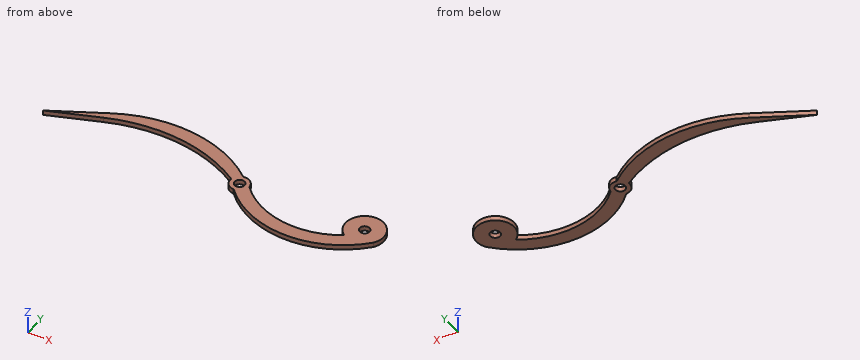
from build123d import *

# Parameters (mm, degrees)
F0_R     = 1.651
F1_DEPTH = 1.6002


with BuildPart() as f1:
    # F0 (on Top) → F1 (new body)
    with BuildSketch(Plane.XY):
        with BuildLine():
            ThreePointArc((-3.774051, -5.106764), (-21.934308, -8.777509), (-38.227296, 0.043366))
            ThreePointArc((-38.227296, 0.043366), (-39.403324, 2.466965), (-42.018165, 3.114637))
            ThreePointArc((-42.018165, 3.114637), (-64.733422, 13.156228), (-89.188089, 8.82198))
            Line((-89.188089, 8.82198), (-106.5022, 0))
            Line((-106.5022, 0), (-90.018623, 5.999531))
            ThreePointArc((-90.018623, 5.999531), (-66.625194, 8.705331), (-44.525194, 0.571215))
            ThreePointArc((-44.525194, 0.571215), (-43.86651, -2.001703), (-41.483321, -3.173958))
            ThreePointArc((-41.483321, -3.173958), (-18.287164, -13.645991), (5.147266, -3.718622))
            ThreePointArc((5.147266, -3.718622), (-0.976301, 6.274499), (-3.774051, -5.106764))
        make_face()
        with Locations((-41.402, 0)):
            Circle(F0_R, mode=Mode.SUBTRACT)
        Circle(F0_R, mode=Mode.SUBTRACT)
    extrude(amount=F1_DEPTH)


solid = f1.part
Geometry check sheet. Reference: the model listing, model coordinates, mm. Coordinates: 2 decimals unless noted, no trailing zeros. Loops run counter-clockwise (first coordinate to the right, second up) from the corner with the lowest first, then second, coordinate; pieces in that order, holes last. Notation, with made-up numbers: (87.25, 22.25) - (138.25, 22.25) arc R32 cw to (138.25, 49.25) - close; hole circle Ø7 at (30.5, -9.75). An arc over 180 degrees is marked (long way). Use one line per item in the form item = value. Start each with the question number.
Item 1: Thickness scan on probe 1 along X at (y, z) = (-1.5, 0.8); probe 2 along Y at (x, z) = (0, 0.7); probe 3 along Y at (x, z) = (-77.5, 0.9). Record the ranges inside material, lowest first.
Item 2: Gauge pin test, flat ends, axial feed: pin 1 (4.5 mm diameter, centred on x = 0, y = 0, fed in from +Z); pin 2 (2 mm diameter, centred on x = -41.402, y = 0, fed in from -Z) (3 decimals). Record the tip position at first contact, or that the pin passes through.
Item 3: Section check D-D, the plane x = -64. Enter the section's corners in (y, z), and give its area (3 significant figures).
Item 4: Section check A-A, the plane x = 0. Enter the section's corners in (y, z).
Item 5: Section check C-C, the plane x = -22.5. Enter the section's corners in (y, z).
Item 6: Section check B-B, the plane z = 0.5. Enter the section's corners in (x, y) (3 decimals), and give its area (3 significant figures).
Computed:
q1.probe_1 = -44.2 to -42.09, -40.71 to -36.74, -6.17 to -0.69, 0.69 to 6.17
q1.probe_2 = -8.11 to -1.65, 1.65 to 6.35
q1.probe_3 = 8.83 to 12.77
q2.pin_1 = 1.6
q2.pin_2 = through
q3.outline = (8.32, 0) - (13.06, 0) - (13.06, 1.6) - (8.32, 1.6) - close
q3.area = 7.58 mm2
q4.outline = (-8.11, 0) - (-1.65, 0) - (-1.65, 1.6) - (-8.11, 1.6) - close; (1.65, 0) - (6.35, 0) - (6.35, 1.6) - (1.65, 1.6) - close
q5.outline = (-13.32, 0) - (-8.69, 0) - (-8.69, 1.6) - (-13.32, 1.6) - close
q6.outline = (-106.502, 0) - (-90.019, 6) arc R50.8 cw to (-44.525, 0.571) arc R3.175 ccw to (-41.483, -3.174) arc R31.75 ccw to (5.147, -3.719) arc R6.35 ccw (long way) to (-3.774, -5.107) arc R27.178 cw to (-38.227, 0.043) arc R3.175 ccw to (-42.018, 3.115) arc R42.596 ccw to (-89.188, 8.822) - close; hole circle Ø3.302 at (-41.402, 0); hole circle Ø3.302 at (0, 0)
q6.area = 552 mm2
